Check sheet for the drawn part. Datum: minimum x, y, z corner. Units: mm. Coordinates: 2 decimals unless noted, no trailing zeros. Order: outer loops, then holes, each group sorted by start corner. A loop starts at its lowest first (then second) coordinate and runs counter-clockwise, first axis right, second up.
1. Cross-section at C-C (y = 11.5). Enter the section's corners in (x, z), then the cut area to 3 significant figures.
2. Cross-section at D-D (x = 1.75). Enter the section's corners in (y, z) (1 decimal).
3. Gauge pin test, flat ends, axial feed: pin 1 Ø0.8 at (x, y) = (15, 32.5) entering from -Z (1 decimal); pin 2 Ø7.5 at (x, z) = (12.5, 2.5) entering from +Y; pin 3 Ø2 at (x, y) = (11, 33.5) entering from +Z (1 decimal); pin 4 Ø12 at (y, z) = (28, 33) entering from -X. Record the tip position at first contact, or that the pin passes through.
4. Cross-section at B-B (y = 2). Enter the section's corners in (x, z).
5. Cross-section at A-A (z = 32.5). Enter the section's corners in (x, y).
6. Thickness scan on line 1 (Z direction, x = 11, y = 10.5); line 2 (Y direction, x = 5.5, z = 32.5); line 3 (X direction, y = 10.5, z = 59.5). Record the ranges inside material, lowest first.
7. Draft check along Y on the marked faces 1, 2 and 3. Enter one of: released by +Y, released by -Y, zero draft, split by the parting line, or undercut.
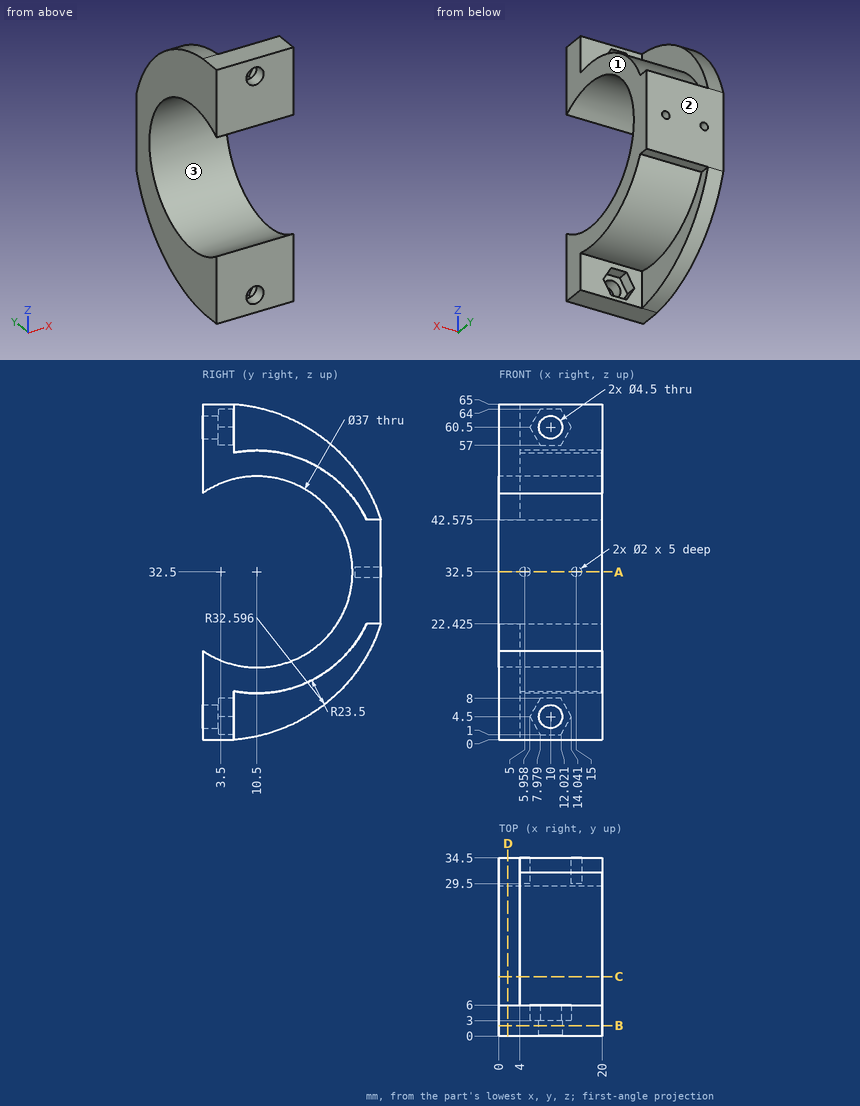
Data:
1. outline: (0, 0.9) - (4, 0.9) - (4, 9.02) - (20, 9.02) - (20, 14.03) - (0, 14.03) - close; (0, 50.97) - (20, 50.97) - (20, 55.98) - (4, 55.98) - (4, 64.1) - (0, 64.1) - close
1. area: 265 mm2
2. outline: (0, 0) - (6, 0) arc R32.6 ccw to (34.5, 22.4) - (34.5, 42.6) arc R32.6 ccw to (6, 65) - (0, 65) - (0, 47.7) arc R18.5 cw (long way) to (0, 17.3) - close
3. pin 1: stops at z = 22.4
3. pin 2: stops at y = 6
3. pin 3: stops at z = 42.6
3. pin 4: stops at x = 0
4. outline: (0, 0) - (20, 0) - (20, 16.07) - (0, 16.07) - close; (0, 48.93) - (20, 48.93) - (20, 65) - (0, 65) - close; hole circle Ø4.5 at (10, 4.5); hole circle Ø4.5 at (10, 60.5)
5. outline: (0, 29) - (20, 29) - (20, 34.5) - (16, 34.5) - (16, 29.5) - (14, 29.5) - (14, 34.5) - (6, 34.5) - (6, 29.5) - (4, 29.5) - (4, 34.5) - (0, 34.5) - close
6. line 1: z = 9 to 14, 51 to 56
6. line 2: y = 29 to 29.5
6. line 3: x = 0 to 4
7. face 1: zero draft
7. face 2: released by +Y
7. face 3: undercut
